```python
from build123d import *

# Parameters (mm, degrees)
SKETCH1_R           = 1.9
BOSS_EXTRUDE1_DEPTH = 10
CIRPATTERN1_COUNT   = 3
CUT_EXTRUDE1_DEPTH  = 10


with BuildPart() as part:
    # Sketch1 → Boss-Extrude1 (new body)
    with BuildSketch(Plane(origin=(0, 0, 0), x_dir=(1, 0, 0), z_dir=(0, 1, 0))):
        with BuildLine():
            ThreePointArc((-2.7961852, 24.843134833), (-6.371318495, 24.174496905), (-9.811597435, 22.99418526))
            Line((-9.811597435, 22.99418526), (-6.639528096, 17.5))
            ThreePointArc((-6.639528096, 17.5), (-5.43375673, 13), (-6.639528096, 8.5))
            Line((-6.639528096, 8.5), (-17.320508076, -10))
            Line((-17.320508076, -10), (17.320508076, -10))
            Line((17.320508076, -10), (-2.7961852, 24.843134833))
        make_face()
        with Locations(Location((0, 0, 0), (0, 0, 270))):
            Circle(SKETCH1_R, mode=Mode.SUBTRACT)
    boss_extrude1 = extrude(amount=BOSS_EXTRUDE1_DEPTH)

    # CirPattern1: Boss-Extrude1 ×3 about axis
    cirpattern1_axis = Axis((0, 0, 0), (0, 1, 0))
    for i in range(1, CIRPATTERN1_COUNT):
        add(boss_extrude1.rotate(cirpattern1_axis, i * 360 / CIRPATTERN1_COUNT))

    # Sketch3 → Cut-Extrude1 (cut)
    with BuildSketch(Plane(origin=(0, 10, 0), x_dir=(1, 0, 0), z_dir=(0, 1, 0))):
        Polygon((3.75277675, 6.5), (-3.75277675, 6.5), (-7.505553499, 0), (-3.75277675, -6.5), (3.75277675, -6.5), (7.505553499, 0), align=None)
    extrude(amount=-CUT_EXTRUDE1_DEPTH, mode=Mode.SUBTRACT)

    # Sketch5 → Cut-Revolve2 (revolve, cut)
    with BuildSketch(Plane.XY, mode=Mode.PRIVATE) as cut_revolve2_sk:
        Polygon((8, 10), (29.75960594, 10), (29.75960594, 3), (9, 3), align=None)
    revolve(cut_revolve2_sk.sketch.rotate(Axis((0, 0, 0), (0, 1, 0)), 90), axis=Axis((0, 0, 0), (0, 1, 0)), mode=Mode.SUBTRACT)


solid = part.part
```
Part model, mm, in its own coordinate system. A direction names the side the tool comes from. Round coordinates to 2 decimals unless told otherwise and drop trailing zeros. Write each loop counter-clockwise with the first axis right and the second up, starting at its lowest first coordinate (ties: lowest second). Pieces come first, ordered by that corner, then holes. Notation, with made-up numbers: (78, 79.5) -> (125, 79.5) arc R31 cw to (125, 104.5) -> close; hole circle Ø8 at (58, -23.75). An arc over 180 degrees is marked (long way). Return JSON: item names as keys, results as strings. Group by question number.
Q1. Which spindle directions (+Z, -Z, +X, -X, +Y, -Y) get a long thin tool onto all of the face, cutting with end or side? Do faces 1 (the flat face through (22, 1, 3)), 2 (the flat face through (5.6, 5.1, 3.3)), 3 (the flat face through (9, 3, -2)). Say none if no direction does.
Q2. Saw through at C-C on z = -11.5. Write the cut outline in (x, y).
Q3. Saw through at A-A on y = 8.25. Write the cut outline in (x, z), plus the area to 3 significant figures.
Q4. Saw through at D-D on x = -16. Write the cut outline in (y, z), plus the area to 3 significant figures.
Q5. Probe L1, parallel to Z at x = -5.5, y = 3.5; L2, parallel to X at y = 3.75, z = 4.5; L3, parallel to X at y = 4.5, z = -3.5. List the from-to ranges inside material, lowest first. Write a range as [from, to].
Q6. Mould opens along X. For faces 4 (the flat face through (-8.25, 1.48, -20.29)), 5 (the flat face through (-5.6, 5.1, -3.3)), 6 (the cylindrical face through (14.032, 1.479, 1.827)) say: pulls with the +X half, pulls with the -X half, needs draft (parallel to the pull), parting line crosses it, or undercut.
Q7. Saw through at B-B on y = 4.5. Write the cut outline in (x, z), plus the area to 3 significant figures.
Q8. Pin check, flat tips, straight feed: pin 1 (0.9 mm diameter, centred on x = 7.5, y = 2, fed in from +Z); pin 2 (12 mm diameter, centred on x = 13, z = 7, fed in from -Y); pin 3 (6 mm diameter, centred on x = 14.5, z = 12, fed in from +Y); pin 4 (4 mm diameter, centred on x = 0.5, y = 5.5, fed in from -Z). Stop position of each tip, or through.
Answer:
{
 "1": {"face 1": "-Z, +X, +Y, -Y", "face 2": "+Y, -Y", "face 3": "+Y"},
 "2": {"outline": "(-5.56, 0) -> (4.91, 0) -> (4.91, 3) -> (-5.56, 3) -> close"},
 "3": {"outline": "circle Ø16.5 at (0, 0); hole (-7.51, 0) -> (-3.75, -6.5) -> (3.75, -6.5) -> (7.51, 0) -> (3.75, 6.5) -> (-3.75, 6.5) -> close", "area": "67.5 mm2"},
 "4": {"outline": "(0, 7.71) -> (3, 7.71) -> (3, 19.21) -> (0, 19.21) -> close", "area": "34.5 mm2"},
 "5": {"L1": "[-7.03, -3.47], [3.47, 7.03]", "L2": "[-7.67, -4.91], [4.91, 7.67]", "L3": "[-8.06, -5.48], [5.48, 8.06]"},
 "6": {"face 4": "pulls with the -X half", "face 5": "undercut", "face 6": "pulls with the +X half"},
 "7": {"outline": "circle Ø17.57 at (0, 0); hole (-7.51, 0) -> (-3.75, -6.5) -> (3.75, -6.5) -> (7.51, 0) -> (3.75, 6.5) -> (-3.75, 6.5) -> close", "area": "96.1 mm2"},
 "8": {"pin 1": "z = 10", "pin 2": "y = 0", "pin 3": "y = 3", "pin 4": "z = -8.92"}
}
